from build123d import *

# Parameters (mm, degrees)
SKETCH1_R           = 17.2
BOSS_EXTRUDE1_DEPTH = 70
SKETCH2_R           = 14
CUT_EXTRUDE1_DEPTH  = 14
SKETCH3_R           = 8.25
CUT_EXTRUDE2_DEPTH  = 50
SKETCH5_R           = 4
BOSS_EXTRUDE2_DEPTH = 10.5
SKETCH9_R           = 16.379462193
BOSS_EXTRUDE4_DEPTH = 4
CUT_EXTRUDE3_START  = -5
CUT_EXTRUDE3_DEPTH  = 50
FILLET2_R           = 2.4
SKETCH7_R           = 6
BOSS_EXTRUDE3_DEPTH = 1
CUT_EXTRUDE4_START  = -2
SKETCH8_R           = 4.26334812
SKETCH8_R_2         = 3.175
CUT_EXTRUDE4_DEPTH  = 0.74
SKETCH10_W          = 4.8
SKETCH10_H          = 4
CUT_EXTRUDE5_DEPTH  = 10


with BuildPart() as part:
    # Sketch1 → Boss-Extrude1 (new body)
    with BuildSketch(Plane.XY):
        Circle(SKETCH1_R)
    extrude(amount=BOSS_EXTRUDE1_DEPTH)

    # Sketch2 → Cut-Extrude1 (cut)
    with BuildSketch(Plane(origin=(0, 0, 0), x_dir=(-1, 0, 0), z_dir=(0, 0, -1))):
        Circle(SKETCH2_R)
    extrude(amount=-CUT_EXTRUDE1_DEPTH, mode=Mode.SUBTRACT)

    # Sketch3 → Cut-Extrude2 (cut)
    with BuildSketch(Plane(origin=(0, 0, 14), x_dir=(-1, 0, 0), z_dir=(0, 0, -1))):
        Circle(SKETCH3_R)
    extrude(amount=-CUT_EXTRUDE2_DEPTH, mode=Mode.SUBTRACT)

    # Sketch4 → Cut-Revolve1 (revolve, cut)
    with BuildSketch(Plane(origin=(0, 0, 0), x_dir=(1, 0, 0), z_dir=(0, 1, 0)), mode=Mode.PRIVATE) as cut_revolve1_sk:
        Polygon((8.25, -64), (0, -66), (0, -64), align=None)
    revolve(cut_revolve1_sk.sketch.rotate(Axis((0, 0, 66), (0, 0, -1)), 180), axis=Axis((0, 0, 66), (0, 0, -1)), mode=Mode.SUBTRACT)

    # Sketch5 → Boss-Extrude2 (add)
    with BuildSketch(Plane.XY.offset(70)):
        with Locations(Location((0, 0, 0), (0, 0, 180))):
            Circle(SKETCH5_R)
    extrude(amount=BOSS_EXTRUDE2_DEPTH)

    # Sketch9 → Boss-Extrude4 (add)
    with BuildSketch(Plane(origin=(0, 0, 14), x_dir=(-1, 0, 0), z_dir=(0, 0, -1))):
        Circle(SKETCH9_R)
        Polygon((-14, 0), (-7, -12.124355653), (7, -12.124355653), (14, 0), (7, 12.124355653), (-7, 12.124355653), align=None, mode=Mode.SUBTRACT)
    extrude(amount=BOSS_EXTRUDE4_DEPTH)

    # Sketch6 → Cut-Extrude3 (cut)
    with BuildSketch(Plane(origin=(0, 0, 0), x_dir=(-1, 0, 0), z_dir=(0, 0, -1)).offset(CUT_EXTRUDE3_START)):
        with BuildLine():
            Line((-2.4, 17.031735085), (-2.4, 12.631735085))
            Line((-2.4, 12.631735085), (2.4, 12.631735085))
            Line((2.4, 12.631735085), (2.4, 17.031735085))
            ThreePointArc((2.4, 17.031735085), (0, 17.2), (-2.4, 17.031735085))
        make_face()
    extrude(amount=-CUT_EXTRUDE3_DEPTH, mode=Mode.SUBTRACT)

    # Fillet2
    fillet2_edges = [part.edges().sort_by_distance(p)[0] for p in [
        (-2.4, 14.831735085, 55),
        (2.4, 14.831735085, 55),
        (-2.4, 15.412243402, 5),
        (2.4, 15.412243402, 5),
    ]]
    fillet(fillet2_edges, radius=FILLET2_R - 0.0001)  # a hair under: the kernel refuses the full size

    # Sketch7 → Boss-Extrude3 (add)
    with BuildSketch(Plane.XY.offset(70)):
        Circle(SKETCH7_R)
    extrude(amount=BOSS_EXTRUDE3_DEPTH)

    # Sketch8 → Cut-Extrude4 (cut)
    with BuildSketch(Plane.XY.offset(80.5).offset(CUT_EXTRUDE4_START)):
        Circle(SKETCH8_R)
        Circle(SKETCH8_R_2, mode=Mode.SUBTRACT)
    extrude(amount=-CUT_EXTRUDE4_DEPTH, mode=Mode.SUBTRACT)

    # Sketch10 → Cut-Extrude5 (cut)
    with BuildSketch(Plane.XZ.offset(-12.124355653)):
        with Locations((0, 12)):
            Rectangle(SKETCH10_W, SKETCH10_H)
    extrude(amount=-CUT_EXTRUDE5_DEPTH, mode=Mode.SUBTRACT)


solid = part.part
Work out the finished part from the listing and answer in its coordinate system (mm). A direction names the side the tool comes from. Give positions to 0.01 mm unless a question says otherwise; leave off trailing zeros. Write each loop counter-clockwise with the first axis right and the second up, starting at its lowest first coordinate (ties: lowest second). Pieces come first, ordered by that corner, then holes. Notation, with made-up numbers: M 36,61 L 42,61 A22 cw 42,80 Z; hole C 9.25,-25.5 d6. An arc over 180 degrees is marked long. Answer as CSV lines item,"result".
Q1. A cutting plane is placed at C-C on x = 10. Write down the section's boundary in (y, z).
A:
outline,"M -13.99,0 L -9.8,0 L -9.8,10 L -6.93,10 L -6.93,14 L 6.93,14 L 6.93,10 L 9.8,10 L 9.8,0 L 13.99,0 L 13.99,70 L -13.99,70 Z"
Q2. Find the intervals of material crossed by probe 1 along Y at (x, z) = (0, 3); probe 2 along Z at (x, y) = (-3, -16); probe 3 along Z at (x, y) = (5, -11.5), in increasing order. Write a range as [from, to].
A:
probe 1,"y = [-17.2, -14], [14, 17.2]"
probe 2,"z = [0, 70]"
probe 3,"z = [14, 70]"
Q3. Given P1, Ø2, axis at x = -11, y = -8, coming from the -Z side; P2, Ø3, axis at y = -5.5, z = 31, coming from the +X side; P3, Ø10, axis at y = -7.5, z = 38, coming from the -X side; P4, Ø5.5, axis at x = -1, z = 36, coming from the +Y side, each flat-ended and moving along its own axis, determine where each tip first touches the part or whether it passes through.
A:
P1,"stops at z = 0"
P2,"stops at x = 16.73"
P3,"stops at x = -17.02"
P4,"stops at y = 17.03"
Q4. A cutting plane is placed at D-D on y = -15. Write down the section's boundary in (x, z), plus the area to 3 significant figures.
A:
outline,"M -8.42,0 L 8.42,0 L 8.42,70 L -8.42,70 Z"
area,"1,180 mm²"
Q5. A tool of negligible diameter and unlimited length cuts with its end or side. For faces 5 (the flat face through (-4, 13, 10)), 6 (the flat face through (0, -7, 70)), 7 (the flat face through (0, 0, 80.5)), 8 (the cylindrical face through (1.716, 14.884, 54.278)), from which of +Z, -Z, +X, -X, +Y, -Y can it reach the whole face along a straight path? Write none if from no direction.
A:
face 5,"-Z"
face 6,"+Z"
face 7,"+Z, +X, -X, +Y, -Y"
face 8,"+Y"
Q6. A cutting plane is placed at A-A on z = 27.5. Write down the section's boundary in (x, y), plus the area to 3 significant figures.
A:
outline,"M -2.4,12.63 L -2.4,17.03 A17.2 ccw long 2.4,17.03 L 2.4,12.63 Z; hole C 0,0 d16.5"
area,"694 mm²"
Q7. The mould has two halves that part along Y. Classify faces 1 (the flat face through (11, -6, 10)), 2 (the flat face through (2.4, 15, 30)), 3 (the flat face through (-10.45, -6.15, 12.03)), 4 (the flat face through (0, 12.632, 34)): +Y half, -Y half, draft (parallel to the pull), parting line (faces both ways), or undercut.
A:
face 1,"undercut"
face 2,"draft"
face 3,"undercut"
face 4,"+Y half"
Q8. A cutting plane is placed at B-B on y = 10. Write down the section's boundary in (x, z), plus the area to 3 significant figures.
A:
outline,"M -13.99,0 L -9.8,0 L -9.8,10 L -8.23,10 L -8.23,14 L 8.23,14 L 8.23,10 L 9.8,10 L 9.8,0 L 13.99,0 L 13.99,70 L -13.99,70 Z"
area,"1,700 mm²"
